Build history of the part. All positions in model axes, mm. A direction names the side the tool comes from. Give positions to 0.01 mm unless a question says otherwise; leave off trailing zeros. Loops run counter-clockwise (first coordinate to the right, second up) from the corner with the lowest first, then second, coordinate; pieces in that order, holes last. Notation, with made-up numbers: (29, 67) -> (72, 67) arc R19 cw to (72, 86) -> close; hole circle Ø5 at (29, 83). An arc over 180 degrees is marked (long way). Answer as a JSON object with one key per item and string values. Group by question number.
Q1. Tool access for faces 1 (the cylindrical face through (20.651, 65.575, -63.031)), 2 (the flat face through (25, -8, -14.482)), 3 (the cylindrical face through (-79.845, 41.53, -86.877)): list every direction of +Z, -Z, +X, -X, +Y, -Y with a clear straight run to the whole face (end or side of a thin tool).
Q2. Two-plate mould, pull along Y, no slides. Class faces 4 (the flat face through (-30, 32, -59.482)), 5 (the cylindrical face through (-92.74, -20.59, -93)), 6 (the cylindrical face through (19.87, 63.095, -77.707)): pulls with the +Y half, pulls with the -Y half, needs draft (parallel to the pull), parting line crosses it, or undercut.
Q3. Band-saw the part on A-A, the plane z = -50.5. Write the cut outline in (x, y), plus the area to 3 significant figures.
Q4. Band-saw the part on B-B, the plane z = -33. Write the cut outline in (x, y).
Q5. Wall check: probe 1 along X at (y, z) = (0, -78); probe 2 along Z at (x, y) = (91, 9); probe 3 along Z at (x, y) = (-77, 77). Give the ranges that are in metal, low to high. Write a range as from..to.
Q6. Drop flat-ended pins along their axis: pin 1 (6 mm diameter, centred on x = 41.5, y = -35, fed in from -Z); pin 2 (8 mm diameter, centred on x = -56.5, z = -66, fed in from -Y); pin 3 (5 mm diameter, centred on y = 77, z = -80, fed in from -X). Give the stop position or say it passes through.
from build123d import *


with BuildPart() as part:
    # Эскиз1 → Повернуть2 (revolve)
    with BuildSketch(Plane(origin=(0, 0, 0), x_dir=(0, 0, -1), z_dir=(1, 0, 0))):
        with BuildLine():
            Line((65.481855233, 20.76), (15.978837376, 23.904897605))
            Line((15.978837376, 23.904897605), (14.481855233, 25.604987877))
            Line((14.481855233, 25.604987877), (14.481855233, 36.5))
            Line((14.481855233, 36.5), (14.981855233, 37))
            Line((14.981855233, 37), (54.481855233, 37))
            ThreePointArc((54.481855233, 37), (58.017389139, 38.464466094), (59.481855233, 42))
            Line((59.481855233, 42), (59.481855233, 68.75))
            Line((59.481855233, 68.75), (66.481855233, 68.75))
            Line((66.481855233, 68.75), (66.481855233, 95.25))
            Line((66.481855233, 95.25), (76.481855233, 105.25))
            Line((76.481855233, 105.25), (81.481855233, 105.25))
            Line((81.481855233, 105.25), (81.481855233, 125))
            Line((81.481855233, 125), (91.481855233, 125))
            Line((91.481855233, 125), (91.481855233, 95))
            Line((91.481855233, 95), (94.481855233, 95))
            Line((94.481855233, 95), (94.481855233, 90))
            Line((94.481855233, 90), (79.481855233, 90))
            Line((79.481855233, 90), (79.481855233, 66.15))
            Line((79.481855233, 66.15), (75.981855233, 66.15))
            Line((75.981855233, 66.15), (75.981855233, 53.186533479))
            Line((75.981855233, 53.186533479), (65.481855233, 35))
            Line((65.481855233, 35), (65.481855233, 20.76))
        make_face()
    revolve(axis=Axis((0, 0, -5.281550862), (0, 0, -1)))


solid = part.part
Worked answers:
{
 "1": {"face 1": "+Z", "face 2": "+Z, +X, -X, +Y, -Y", "face 3": "-Z"},
 "2": {"face 4": "needs draft", "face 5": "parting line crosses it", "face 6": "undercut"},
 "3": {"outline": "circle Ø74 at (0, 0); hole circle Ø43.42 at (0, 0)", "area": "2,820 mm2"},
 "4": {"outline": "circle Ø74 at (0, 0); hole circle Ø45.65 at (0, 0)"},
 "5": {"probe 1": "-105.25..-66.15, 66.15..105.25", "probe 2": "-94.48..-66.48", "probe 3": "-91.48..-81.48"},
 "6": {"pin 1": "z = -75.98", "pin 2": "y = -81.73", "pin 3": "x = -100.01"}
}
